Geometry check sheet. Reference: the model listing, model coordinates, mm. Face numbers are marked on the shaded views. A direction names the side the tool comes from. Coordinates: 2 decimals unless noted, no trailing zeros. Write each loop counter-clockwise with the first axis right and the second up, starting at its lowest first coordinate (ties: lowest second). Pieces come first, ordered by that corner, then holes. Notation, with made-up numbers: (-26, -14.5) -> (30, -14.5) arc R6 ccw to (30, -9.5) -> close; hole circle Ø8 at (-0.5, 2.25). An arc over 180 degrees is marked (long way). Answer in a Markdown table with one row per item. Add a question column.
1. Cross-section at B-B on z = 5.25. Record the cut outline in (x, y).
2. Scan lines: L1, parallel to X at y = 14.5, z = 2; L2, parallel to X at y = 14.75, z = 2.75; L3, parallel to Z at x = 13, y = 13.25. Record each from-to range of solid material in increasing order. Write a range as from..to.
3. Set-up check for the marked faces 3, 4 and 5: record each of +Z, -Z, +X, -X, +Y, -Y from which the full face is reachable in a straight line by a thin tool's end or side.
4. Cross-section at D-D on y = 20.25. Record the cut outline in (x, z).
5. Depth check by flat-ended pin: P1, Ø2, axis at y = 7.5, z = 6.5, coming from the -X side; P2, Ø4.5, axis at x = 12.5, y = 11.5, coming from the +Z side; P3, Ø2, axis at x = 1, z = 4.5, coming from the -Y side. Enter the tip coordinate at first touch or a pass-through.
6. Cross-section at C-C on x = 9.6. Record the cut outline in (y, z), and give its area (3 significant figures).
7. Mould release check, pull along X, two halves, no side actions. Record for the marked faces 1 and 2: pulls with the +X half, pulls with the -X half, needs draft (parallel to the pull), parting line crosses it, or undercut.
8. Cross-section at A-A on y = 9.75. Record the cut outline in (x, z).
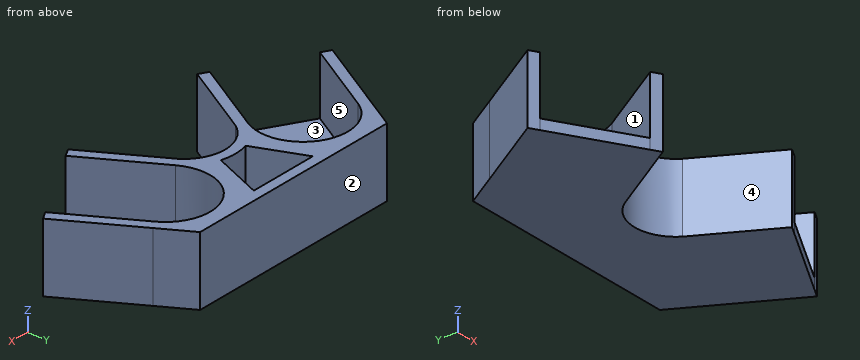
```python
from build123d import *

# Parameters (mm, degrees)
F1_DEPTH = 1.2
F3_DEPTH = 8
F5_DEPTH = 6.8


with BuildPart() as f1:
    # F0 (on Top) → F1 (new body)
    with BuildSketch(Plane.XY):
        with BuildLine():
            Line((-19.146633, 10.592434), (-10.053367, 5.342434))
            Line((-10.053367, 5.342434), (-5.053367, 14.002688))
            ThreePointArc((-5.053367, 14.002688), (0, 16.767957), (5.053367, 14.002688))
            Line((5.053367, 14.002688), (10.053367, 5.342434))
            Line((10.053367, 5.342434), (19.146633, 10.592434))
            Line((19.146633, 10.592434), (14.146633, 19.252688))
            Line((14.146633, 19.252688), (12.342414, 22.377688))
            Line((12.342414, 22.377688), (-12.342414, 22.377688))
            Line((-12.342414, 22.377688), (-14.146633, 19.252688))
            Line((-14.146633, 19.252688), (-19.146633, 10.592434))
        make_face()
    extrude(amount=F1_DEPTH)

    # F2 (on face) → F3 (join)
    with BuildSketch(Plane.XY):
        with BuildLine():
            Line((-5.053367, 14.002688), (-10.053367, 5.342434))
            Line((-10.053367, 5.342434), (-9.014136, 4.742434))
            Line((-9.014136, 4.742434), (-4.024356, 13.384986))
            ThreePointArc((-4.024356, 13.384986), (0, 15.568776), (4.024356, 13.384986))
            Line((4.024356, 13.384986), (9.014136, 4.742434))
            Line((9.014136, 4.742434), (10.053367, 5.342434))
            Line((10.053367, 5.342434), (5.053367, 14.002688))
            ThreePointArc((5.053367, 14.002688), (0, 16.767957), (-5.053367, 14.002688))
        make_face()
        Polygon((-19.146633, 10.592434), (-14.146633, 19.252688), (-12.342414, 22.377688), (12.342414, 22.377688), (14.146633, 19.252688), (19.146633, 10.592434), (20.185864, 11.192434), (15.185864, 19.852688), (13.035234, 23.577688), (-13.035234, 23.577688), (-15.185864, 19.852688), (-20.185864, 11.192434), align=None)
    extrude(amount=F3_DEPTH)

    # F4 (on face) → F5 (join, through all)
    with BuildSketch(Plane.XY.offset(1.2)):
        with BuildLine():
            Line((-4.113592, 22.377688), (-12.342414, 22.377688))
            Line((-12.342414, 22.377688), (-14.146633, 19.252688))
            ThreePointArc((-14.146633, 19.252688), (-6.975, 21.174321), (-5.053367, 14.002688))
            ThreePointArc((-5.053367, 14.002688), (-3.614694, 15.556901), (-1.725656, 16.514443))
            Line((-1.725656, 16.514443), (-4.113592, 22.377688))
        make_face()
        with BuildLine():
            ThreePointArc((1.725656, 16.514443), (3.614694, 15.556901), (5.053367, 14.002688))
            ThreePointArc((5.053367, 14.002688), (6.975, 21.174321), (14.146633, 19.252688))
            Line((14.146633, 19.252688), (12.342414, 22.377688))
            Line((12.342414, 22.377688), (4.113592, 22.377688))
            Line((4.113592, 22.377688), (1.725656, 16.514443))
        make_face()
    extrude(amount=F5_DEPTH)


solid = f1.part
```
Results found:
| question | item | result |
|---|---|---|
| 1 | outline | (-20.19, 11.19) -> (-19.15, 10.59) -> (-14.15, 19.25) arc R5.25 cw to (-5.05, 14) -> (-10.05, 5.34) -> (-9.01, 4.74) -> (-4.02, 13.38) arc R4.8 cw to (4.02, 13.38) -> (9.01, 4.74) -> (10.05, 5.34) -> (5.05, 14) arc R5.25 cw to (14.15, 19.25) -> (19.15, 10.59) -> (20.19, 11.19) -> (13.04, 23.58) -> (-13.04, 23.58) -> close; hole (-4.11, 22.38) -> (-1.73, 16.51) arc R6 cw to (1.73, 16.51) -> (4.11, 22.38) -> close |
| 2 | L1 | x = -18.28..-16.89, -4.8..-3.02, 3.02..4.8, 16.89..18.28 |
| 2 | L2 | x = -18.13..-16.75, -4.7..-2.68, 2.68..4.7, 16.75..18.13 |
| 2 | L3 | z = 0..1.2 |
| 3 | face 3 | +Z |
| 3 | face 4 | +Z, -Z, -Y |
| 3 | face 5 | +Z, -Y |
| 4 | outline | (-14.96, 0) -> (14.96, 0) -> (14.96, 8) -> (13.4, 8) -> (13.4, 1.2) -> (5.8, 1.2) -> (5.8, 8) -> (3.25, 8) -> (3.25, 1.2) -> (-3.25, 1.2) -> (-3.25, 8) -> (-5.8, 8) -> (-5.8, 1.2) -> (-13.4, 1.2) -> (-13.4, 8) -> (-14.96, 8) -> close |
| 5 | P1 | stops at x = -9.39 |
| 5 | P2 | stops at z = 1.2 |
| 5 | P3 | stops at y = 15.13 |
| 6 | outline | (5.08, 0) -> (23.58, 0) -> (23.58, 8) -> (21.88, 8) -> (21.88, 1.2) -> (6.13, 1.2) -> (6.13, 8) -> (5.08, 8) -> close |
| 6 | area | 40.9 mm^2 |
| 7 | face 1 | undercut |
| 7 | face 2 | needs draft |
| 8 | outline | (-17.69, 0) -> (-6.12, 0) -> (-6.12, 8) -> (-7.51, 8) -> (-7.51, 1.2) -> (-17.69, 1.2) -> close; (6.12, 0) -> (17.69, 0) -> (17.69, 1.2) -> (7.51, 1.2) -> (7.51, 8) -> (6.12, 8) -> close |
